Check sheet for the modelled part. Datum: model origin and axes. Units: mm. Face numbers are marked on the shaded views. A direction names the side the tool comes from. Coordinates: 2 decimals unless noted, no trailing zeros. Write each loop counter-clockwise with the first axis right and the second up, starting at its lowest first coordinate (ties: lowest second). Pieces come first, ordered by that corner, then holes. Notation, with made-up numbers: (63.25, 44) - (98.25, 44) arc R20 cw to (98.25, 64) - close; hole circle Ø2 at (-22.5, -20). An arc over 180 degrees is marked (long way). Use one line per item in the form item = value. Start each with the question number.
1. Tool access check on the marked faces 4, 5 and 6. Record the directions out of +Z, -Z, +X, -X, +Y, -Y that give a thin tool (end or side, any length) a straight path to the whole face; none if there is none.
2. Scan lines: line 1 along X through (y, z) = (3.2, 0); line 2 along X through (y, z) = (-0.4, 0); line 3 along Y through (x, z) = (1, -1.5). Record each from-to range of solid material in increasing order.
3. Go/stop test with flat-tipped pins: pin 1 Ø4 at (x, z) = (0, 0) entering from -Y; pin 2 Ø1.5 at (x, y) = (-1, 3) entering from +Z; pin 3 Ø1 at (y, z) = (0, -1.5) entering from -X. Record where each tip stops, or that it passes through.
4. Draft check along Z on the marked faces 1, 2 and 3. Enter one of: +Z half, -Z half, draft (parallel to the pull), parting line (faces both ways), or undercut.
5. Cross-section at C-C on y = -0.3. Record the boundary of the cut face in (x, z).
```python
from build123d import *

# Parameters (mm, degrees)
SKETCH1_R           = 3.9878
BOSS_EXTRUDE1_DEPTH = 1.6256
SKETCH2_R           = 4.0005
BOSS_EXTRUDE2_DEPTH = 2.54
SKETCH3_R           = 3.5179
BOSS_EXTRUDE3_DEPTH = 0.762
SKETCH4_R           = 3.0099
CUT_EXTRUDE1_DEPTH  = 0.762
SKETCH5_R           = 2.6289
CUT_EXTRUDE2_DEPTH  = 2.54
SKETCH6_R           = 1.397
CUT_EXTRUDE3_DEPTH  = 7.201580484


with BuildPart() as part:
    # Sketch1 → Boss-Extrude1 (new body)
    with BuildSketch(Plane(origin=(0, 0, 0), x_dir=(1, 0, 0), z_dir=(0, 1, 0))):
        with Locations(Location((0, 0, 0), (0, 0, 270))):
            Circle(SKETCH1_R)
    extrude(amount=BOSS_EXTRUDE1_DEPTH)

    # Sketch2 → Boss-Extrude2 (add)
    with BuildSketch(Plane(origin=(0, 1.6256, 0), x_dir=(1, 0, 0), z_dir=(0, 1, 0))):
        with Locations(Location((0, 0, 0), (0, 0, 270))):
            Circle(SKETCH2_R)
    extrude(amount=BOSS_EXTRUDE2_DEPTH)

    # Sketch3 → Boss-Extrude3 (add)
    with BuildSketch(Plane.XZ):
        with Locations(Location((0, 0, 0), (0, 0, 90))):
            Circle(SKETCH3_R)
    extrude(amount=BOSS_EXTRUDE3_DEPTH)

    # Sketch4 → Cut-Extrude1 (cut)
    with BuildSketch(Plane.XZ.offset(0.762)):
        with Locations(Location((0, 0, 0), (0, 0, 270))):
            Circle(SKETCH4_R)
    extrude(amount=-CUT_EXTRUDE1_DEPTH, mode=Mode.SUBTRACT)

    # Sketch5 → Cut-Extrude2 (cut)
    with BuildSketch(Plane(origin=(0, 4.1656, 0), x_dir=(1, 0, 0), z_dir=(0, 1, 0))):
        with Locations(Location((0, 0, 0), (0, 0, 270))):
            Circle(SKETCH5_R)
    extrude(amount=-CUT_EXTRUDE2_DEPTH, mode=Mode.SUBTRACT)

    # Sketch6 → Cut-Extrude3 (cut, through all)
    with BuildSketch(Plane(origin=(0, 1.6256, 0), x_dir=(1, 0, 0), z_dir=(0, 1, 0))):
        with Locations(Location((0, 0, 0), (0, 0, 270))):
            Circle(SKETCH6_R)
    extrude(amount=-CUT_EXTRUDE3_DEPTH, mode=Mode.SUBTRACT)


solid = part.part
```
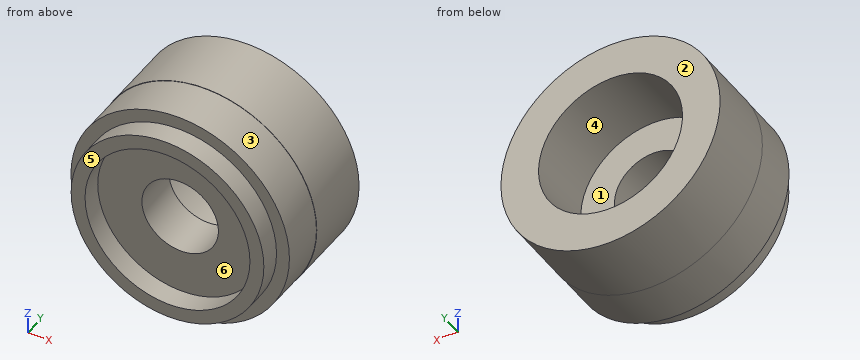
Final values:
q1.face_4 = +Y
q1.face_5 = +Z, -Z, +X, -X, -Y
q1.face_6 = -Y
q2.line_1 = -4 to -2.63, 2.63 to 4
q2.line_2 = -3.52 to -3.01, 3.01 to 3.52
q2.line_3 = 0 to 1.63
q3.pin_1 = 0
q3.pin_2 = 3.99
q3.pin_3 = -3.86
q4.face_1 = undercut
q4.face_2 = draft
q4.face_3 = parting line
q5.outline = circle Ø7.04 at (0, 0); hole circle Ø6.02 at (0, 0)
